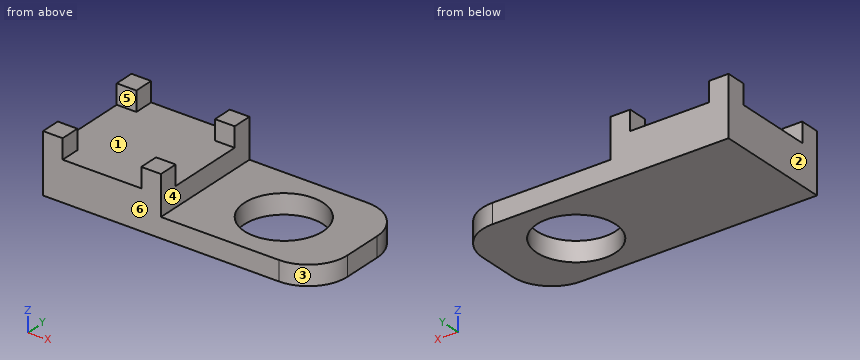
Autodesk Fusion 360 part; units mm, degrees
sketch "Sketch1" plane through (0, 0, 0) normal (0, 0, 1) x (1, 0, 0)
  line L0 (62.7035, 16.041) -> (62.7035, 166.041)
  line L1 (62.7035, 16.041) -> (362.7035, 16.041)
  line L2 (62.7035, 166.041) -> (362.7035, 166.041)
  line L3 (412.7035, 116.041) -> (412.7035, 66.041)
  arc A0 (412.7035, 116.041) -> (362.7035, 166.041) centre (362.7035, 116.041) ccw
  arc A1 (362.7035, 16.041) -> (412.7035, 66.041) centre (362.7035, 66.041) ccw
  line L4 (212.7035, 166.041) -> (212.7035, 16.041)
  circle A2 centre (312.7035, 91.041) radius 50
  line L5 (62.7035, 166.041) -> (87.7035, 166.041)
  line L6 (87.7035, 166.041) -> (87.7035, 141.041)
  line L7 (87.7035, 141.041) -> (62.7035, 141.041)
  line L8 (62.7035, 141.041) -> (62.7035, 166.041)
  line L9 (212.7035, 166.041) -> (187.7035, 166.041)
  line L10 (187.7035, 166.041) -> (187.7035, 141.041)
  line L11 (187.7035, 141.041) -> (212.7035, 141.041)
  line L12 (212.7035, 141.041) -> (212.7035, 166.041)
  line L13 (62.7035, 16.041) -> (87.7035, 16.041)
  line L14 (87.7035, 16.041) -> (87.7035, 41.041)
  line L15 (87.7035, 41.041) -> (62.7035, 41.041)
  line L16 (62.7035, 41.041) -> (62.7035, 16.041)
  line L17 (212.7035, 16.041) -> (187.7035, 16.041)
  line L18 (187.7035, 16.041) -> (187.7035, 41.041)
  line L19 (187.7035, 41.041) -> (212.7035, 41.041)
  line L20 (212.7035, 41.041) -> (212.7035, 16.041)
  point P0 (412.7035, 16.041)
  point P1 (412.7035, 166.041)
  dimension "d1" = 150
  dimension "d2" = 350
  dimension "d3" = 350
  dimension "d4" = 50
  dimension "d5" = 50
  dimension "d8" = 100
  dimension "d9" = 25
  dimension "d10" = 25
  dimension "d11" = 25
  dimension "d12" = 25
  dimension "d13" = 25
  dimension "d14" = 25
  dimension "d15" = 25
  dimension "d16" = 25
extrude "Extrude1" add sketch "Sketch1" along normal blind 25 contours L1 L2 L3 A0 A1 L4 L12 L20
extrude "Extrude2" add sketch "Sketch1" along normal blind 50 contours L0 L1 L2 L4 L6 L7 L10 L11 L14 L15 L18 L19
extrude "Extrude3" add sketch "Sketch1" along normal blind 75 contours L0 L1 L13 L14 L15 L16 | L0 L2 L5 L6 L7 L8 | L1 L4 L17 L18 L19 L20 | L2 L4 L9 L10 L11 L12
Build history of the part. All positions in model axes, mm. Face numbers are marked on the shaded views. A direction names the side the tool comes from. Coordinates: 2 decimals unless noted, no trailing zeros. Order: outer loops, then holes, each group sorted by start corner. A loop starts at its lowest first (then second) coordinate and runs counter-clockwise, first axis right, second up. Notation, with made-up numbers: (-28.75, -34.5) -> (-16.75, -34.5) arc R16 ccw to (-16.75, -23.5) -> close; hole circle Ø5 at (49.25, 79.5). An arc over 180 degrees is marked (long way). Answer in a Markdown table with one row per item. Add a question column.
Q1. Band-saw the part on D-D, the plane z = 7. List the corners of the cut face in (x, y).
Q2. Mould opens along X. For the marked faces 1, 2 and 3 say: +X half, -X half, draft (parallel to the pull), parting line (faces both ways), or undercut.
Q3. Band-saw the part on A-A, the plane z = 67. List the corners of the cut face in (x, y), then the cut area to 3 significant figures.
Q4. Band-saw the part on B-B, the plane x = 357. List the corners of the cut face in (y, z), then the cut area to 3 significant figures.
Q5. Band-saw the part on C-C, the plane y = 131. List the corners of the cut face in (x, z), then the cut area to 3 significant figures.
Q6. Which spindle directions (+Z, -Z, +X, -X, +Y, -Y) get a long thin tool onto all of the face, cutting with end or side? Do the marked faces 4, 5 and 6. Say none if no direction does.
Q7. Drop flat-ended pins along their axis: pin 1 (20 mm diameter, centred on y = 33.5, z = 66.5, fed in from +X); pin 2 (1.5 mm diameter, centred on x = 376.5, z = 22.5, fed in from +Y); pin 3 (1 mm diameter, centred on x = 246, y = 76.5, fed in from +Z). Give the stop position or say it passes through.
Q8. Wall check: line 1 along X through (y, z) = (153.5, 55.5); line 2 along Z through (x, y) = (173, 40); line 3 along X through (y, z) = (90, 37). Give the ranges that are in metal, low to high. Write a range as [from, to].
Answers follow:
| question | item | result |
|---|---|---|
| 1 | outline | (62.7, 16.04) -> (362.7, 16.04) arc R50 ccw to (412.7, 66.04) -> (412.7, 116.04) arc R50 ccw to (362.7, 166.04) -> (62.7, 166.04) -> close; hole circle Ø100 at (312.7, 91.04) |
| 2 | face 1 | undercut |
| 2 | face 2 | -X half |
| 2 | face 3 | +X half |
| 3 | outline | (62.7, 16.04) -> (87.7, 16.04) -> (87.7, 41.04) -> (62.7, 41.04) -> close; (62.7, 141.04) -> (87.7, 141.04) -> (87.7, 166.04) -> (62.7, 166.04) -> close; (187.7, 16.04) -> (212.7, 16.04) -> (212.7, 41.04) -> (187.7, 41.04) -> close; (187.7, 141.04) -> (212.7, 141.04) -> (212.7, 166.04) -> (187.7, 166.04) -> close |
| 3 | area | 2,500 mm^2 |
| 4 | outline | (16.04, 0) -> (67.85, 0) -> (67.85, 25) -> (16.04, 25) -> close; (114.23, 0) -> (166.04, 0) -> (166.04, 25) -> (114.23, 25) -> close |
| 4 | area | 2,590 mm^2 |
| 5 | outline | (62.7, 0) -> (282.65, 0) -> (282.65, 25) -> (212.7, 25) -> (212.7, 50) -> (62.7, 50) -> close; (342.76, 0) -> (410.41, 0) -> (410.41, 25) -> (342.76, 25) -> close |
| 5 | area | 10,900 mm^2 |
| 6 | face 4 | +Z, +X, +Y, -Y |
| 6 | face 5 | +Z, +X, -X |
| 6 | face 6 | +Z, -Z, +X, -X, -Y |
| 7 | pin 1 | x = 212.7 |
| 7 | pin 2 | y = 164.31 |
| 7 | pin 3 | z = 25 |
| 8 | line 1 | [62.7, 87.7], [187.7, 212.7] |
| 8 | line 2 | [0, 50] |
| 8 | line 3 | [62.7, 212.7] |
